from build123d import *

# Parameters (mm, degrees)
SKETCH_1_R      = 2.5
SKETCH_1_R_2    = 1.5
SKETCH_1_R_3    = 2
EXTRUDE_1_DEPTH = 3


with BuildPart() as part:
    # 草图1 → 凸台-拉伸1 (new body)
    with BuildSketch(Plane.XZ):
        with BuildLine():
            Line((-154.308657865, -118), (-35, -118))
            ThreePointArc((-35, -118), (-31.464466094, -116.535533906), (-30, -113))
            Line((-30, -113), (-30, 113))
            ThreePointArc((-30, 113), (-31.464466094, 116.535533906), (-35, 118))
            Line((-35, 118), (-154.308657865, 118))
            ThreePointArc((-154.308657865, 118), (-155.07402473, 117.847759065), (-155.722871427, 117.414213562))
            Line((-155.722871427, 117.414213562), (-191.379725677, 81.757359313))
            ThreePointArc((-191.379725677, 81.757359313), (-192.680362185, 79.81081922), (-193.13708499, 77.514718626))
            Line((-193.13708499, 77.514718626), (-193.13708499, -77.514718626))
            ThreePointArc((-193.13708499, -77.514718626), (-192.680362185, -79.81081922), (-191.379725677, -81.757359313))
            Line((-191.379725677, -81.757359313), (-155.722871427, -117.414213562))
            ThreePointArc((-155.722871427, -117.414213562), (-155.07402473, -117.847759065), (-154.308657865, -118))
        make_face()
        with Locations(Location((-140, 59.5, 0), (0, 0, 270))):
            Circle(SKETCH_1_R, mode=Mode.SUBTRACT)
        with Locations(Location((-170, -59.5, 0), (0, 0, 270))):
            Circle(SKETCH_1_R, mode=Mode.SUBTRACT)
        with Locations(Location((-140, -59.5, 0), (0, 0, 270))):
            Circle(SKETCH_1_R, mode=Mode.SUBTRACT)
        with Locations(Location((-178.13708499, 60, 0), (0, 0, 270))):
            Circle(SKETCH_1_R, mode=Mode.SUBTRACT)
        with Locations(Location((-178.13708499, -60, 0), (0, 0, 270))):
            Circle(SKETCH_1_R, mode=Mode.SUBTRACT)
        with Locations(Location((-168.388347648, -83.535533906, 0), (0, 0, 270))):
            Circle(SKETCH_1_R, mode=Mode.SUBTRACT)
        with Locations(Location((-168.388347648, 83.535533906, 0), (0, 0, 270))):
            Circle(SKETCH_1_R, mode=Mode.SUBTRACT)
        with Locations(Location((-45, -45, 0), (0, 0, 270))):
            Circle(SKETCH_1_R_2, mode=Mode.SUBTRACT)
        with Locations(Location((-45, 45, 0), (0, 0, 270))):
            Circle(SKETCH_1_R_2, mode=Mode.SUBTRACT)
        with Locations(Location((-36, -40, 0), (0, 0, 270))):
            Circle(SKETCH_1_R, mode=Mode.SUBTRACT)
        with Locations(Location((-36, 40, 0), (0, 0, 270))):
            Circle(SKETCH_1_R, mode=Mode.SUBTRACT)
        with Locations(Location((-62, 84, 0), (0, 0, 270))):
            Circle(SKETCH_1_R, mode=Mode.SUBTRACT)
        with Locations(Location((-90, 84, 0), (0, 0, 270))):
            Circle(SKETCH_1_R, mode=Mode.SUBTRACT)
        with Locations(Location((-113, 84, 0), (0, 0, 270))):
            Circle(SKETCH_1_R, mode=Mode.SUBTRACT)
        with Locations(Location((-62, -84, 0), (0, 0, 270))):
            Circle(SKETCH_1_R, mode=Mode.SUBTRACT)
        with Locations(Location((-90, -84, 0), (0, 0, 270))):
            Circle(SKETCH_1_R, mode=Mode.SUBTRACT)
        with Locations(Location((-113, -84, 0), (0, 0, 270))):
            Circle(SKETCH_1_R, mode=Mode.SUBTRACT)
        with Locations(Location((-100, -108, 0), (0, 0, 270))):
            Circle(SKETCH_1_R, mode=Mode.SUBTRACT)
        with Locations(Location((-100, 108, 0), (0, 0, 270))):
            Circle(SKETCH_1_R, mode=Mode.SUBTRACT)
        with Locations(Location((-139.220192924, 113.764348802, 0), (0, 0, 270))):
            Circle(SKETCH_1_R, mode=Mode.SUBTRACT)
        with Locations(Location((-139.220192924, 82.651650429, 0), (0, 0, 270))):
            Circle(SKETCH_1_R, mode=Mode.SUBTRACT)
        with Locations(Location((-139.220192924, -113.764348802, 0), (0, 0, 270))):
            Circle(SKETCH_1_R, mode=Mode.SUBTRACT)
        with Locations(Location((-139.220192924, -82.651650429, 0), (0, 0, 270))):
            Circle(SKETCH_1_R, mode=Mode.SUBTRACT)
        with Locations(Location((-40, 70, 0), (0, 0, 270))):
            Circle(SKETCH_1_R_3, mode=Mode.SUBTRACT)
        with Locations(Location((-40, -70, 0), (0, 0, 270))):
            Circle(SKETCH_1_R_3, mode=Mode.SUBTRACT)
        with Locations(Location((-40, 0, 0), (0, 0, 270))):
            Circle(SKETCH_1_R_3, mode=Mode.SUBTRACT)
        with Locations(Location((-170, 59.5, 0), (0, 0, 270))):
            Circle(SKETCH_1_R, mode=Mode.SUBTRACT)
        Polygon((-170.156114601, 98.738329701), (-155.306872196, 113.587572106), (-139.39696962, 97.67766953), (-154.246212025, 82.828427125), align=None, mode=Mode.SUBTRACT)
        Polygon((-170.156114601, -98.738329701), (-154.246212025, -82.828427125), (-139.39696962, -97.67766953), (-155.306872196, -113.587572106), align=None, mode=Mode.SUBTRACT)
    extrude(amount=-EXTRUDE_1_DEPTH)


solid = part.part
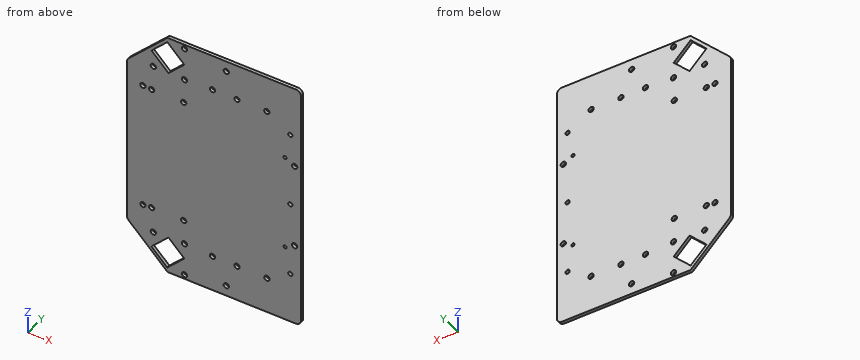
Could you check a few things on this model? Use its own coordinates, in mm. Give positions to 0.01 mm unless a question says otherwise; leave off trailing zeros. Write each loop counter-clockwise with the first axis right and the second up, starting at its lowest first coordinate (ties: lowest second). Pieces come first, ordered by that corner, then holes. Notation, with made-up numbers: (41.5, 55) -> (95.5, 55) arc R6 ccw to (95.5, 62) -> close; hole circle Ø2 at (40.5, 15). An arc over 180 degrees is marked (long way). Answer as CSV lines item,"result". Start each with the question number.
(1) If we section it at B-B, the plane z = 95: Write out the boundary of the cut face in (x, y), and give its area (3 significant figures).
(2) If we section it at A-A, the plane x = -100: Write out the boundary of the cut face in (y, z), and give its area (3 significant figures).
(3) If we section it at D-D, the plane y = 1.8: Give the number of separate pieces and of enclosed holes in the cut face, and give its area (3 significant figures).
(4) I'm going to push a flat-ended pin straight in: pin 1 Ø2.5 at (x, z) = (-40, 70) entering from -Y. Where does the tip first touch, or does it pass through?
(5) If we section it at C-C, the plane z = -108: Write out the boundary of the cut face in (x, y).
(6) Please list where these lines run through material, in increasing order: line 1 (Z direction, x = -178, y = 0.4); line 2 (X direction, y = 2.2, z = -90); line 3 (X direction, y = 1.35, z = -80).
Answer list:
1,outline,"(-178.14, 0) -> (-166.42, 0) -> (-166.42, 3) -> (-178.14, 3) -> close; (-142.07, 0) -> (-30, 0) -> (-30, 3) -> (-142.07, 3) -> close"
1,area,"371 mm^2"
2,outline,"(0, -118) -> (3, -118) -> (3, -110.5) -> (0, -110.5) -> close; (0, -105.5) -> (3, -105.5) -> (3, 105.5) -> (0, 105.5) -> close; (0, 110.5) -> (3, 110.5) -> (3, 118) -> (0, 118) -> close"
2,area,"678 mm^2"
3,separate pieces,"1"
3,enclosed holes,"29"
3,area,"35,600 mm^2"
4,pin 1,"through"
5,outline,"(-165.14, 0) -> (-160.89, 0) -> (-160.89, 3) -> (-165.14, 3) -> close; (-149.72, 0) -> (-102.5, 0) -> (-102.5, 3) -> (-149.72, 3) -> close; (-97.5, 0) -> (-30, 0) -> (-30, 3) -> (-97.5, 3) -> close"
6,line 1,"-95.14 to -62.5, -57.5 to 57.5, 62.5 to 95.14"
6,line 2,"-183.14 to -161.42, -147.07 to -30"
6,line 3,"-192.6 to -30"
